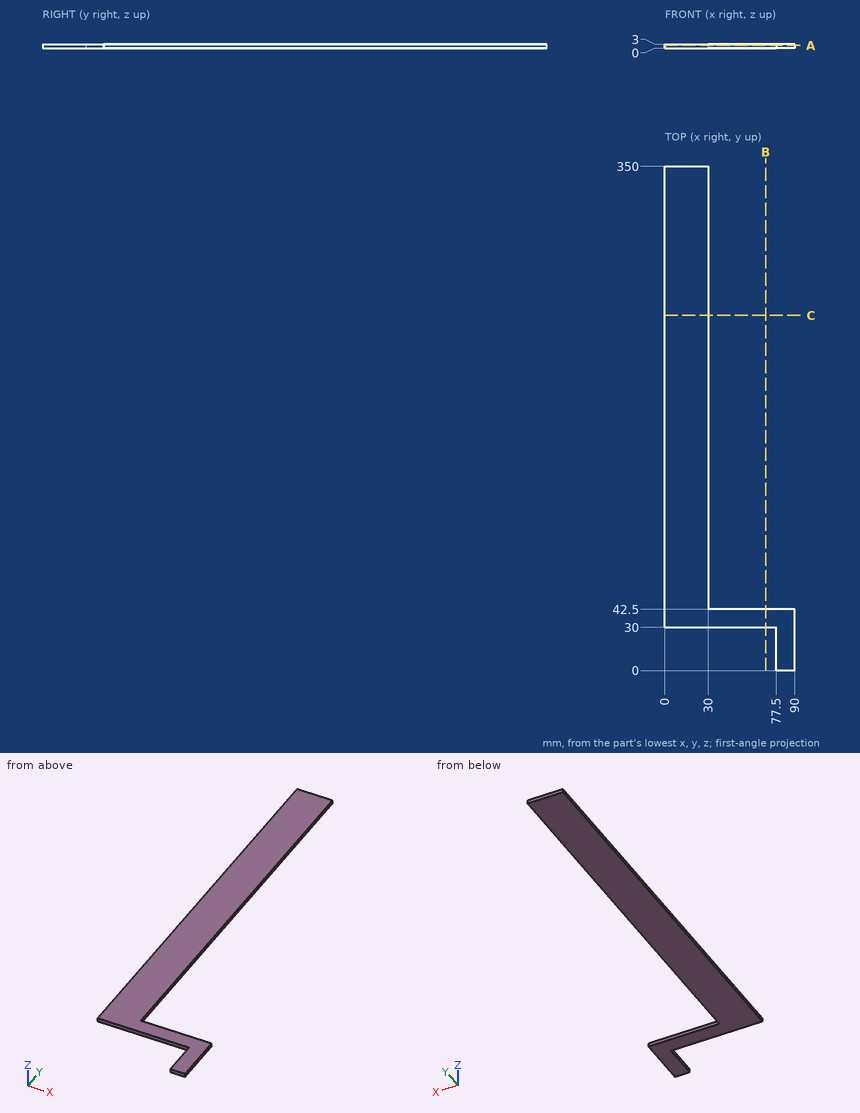
Geometry: see drawing. Coordinates: mm, zero at the bounding-box minimum. Round coordinates to 2 decimals unless told otherwise and drop trailing zeros. Write each loop counter-clockwise with the first axis right and the second up, starting at its lowest first coordinate (ties: lowest second). Pieces come first, ordered by that corner, then holes.
Item 1: Section query B-B (x = 70). Return loops of the section in (y, z), plus the area to 3 significant figures.
Item 2: Pin query (flat end, axial travel): P1, Ø1, axis at x = 44.5, z = 1.5, coming from the -Y side; P2, Ø5, axis at x = 26, y = 40.5, coming from the -Z side; P3, Ø0.9, axis at y = 16, z = 2, coming from the -X side. Return the tip coordinate at first contact, or that it passes through.
Item 3: Material intervals for L1, parallel to Y at x = 70, z = 1.3; L2, parallel to Y at x = 24, z = 2.5; L3, parallel to X at y = 278.5, z = 1.85, sorted ascending.
Item 4: Section query A-A (z = 2). Return loops of the section in (x, y).
Item 5: Section query C-C (y = 246.5). Return loops of the section in (x, z), plus the area to 3 significant figures.
Completed:
1. outline: (30, 0) - (42.5, 0) - (42.5, 3) - (30, 3) - close
1. area: 37.5 mm2
2. P1: stops at y = 30
2. P2: stops at z = 0
2. P3: stops at x = 77.5
3. L1: y = 30 to 42.5
3. L2: y = 30 to 350
3. L3: x = 0 to 30
4. outline: (0, 30) - (77.5, 30) - (77.5, 0) - (90, 0) - (90, 42.5) - (30, 42.5) - (30, 350) - (0, 350) - close
5. outline: (0, 0) - (30, 0) - (30, 3) - (0, 3) - close
5. area: 90.0 mm2
